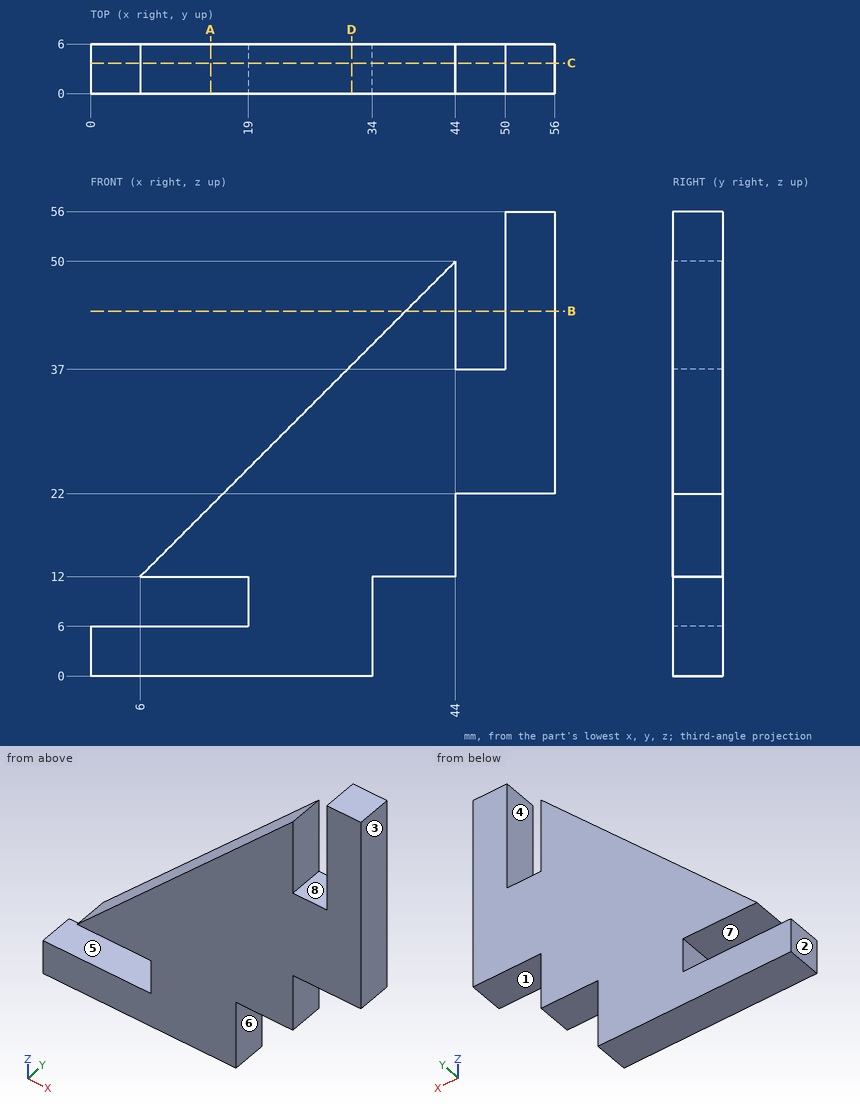
Print and shaded views of the part. All mm, measured from the part's lowest x, y and z. A direction names the side the tool comes from. Coordinates: 2 decimals unless noted, no trailing zeros. Loops run counter-clockwise (first coordinate to the right, second up) from the corner with the lowest first, then second, coordinate; pieces in that order, holes last. Notation, with made-up numbers: (87, 66) - (137, 66) arc R17 ccw to (137, 97) - close; hole circle Ø9 at (72, 30.5). An arc over 180 degrees is marked (long way). Write item = value, one per line. Start each with the question number.
Item 1: Flat gauge pins, fed straight in: pin 1 Ø1.8 at (y, z) = (1.5, 10.5) entering from -X; pin 2 Ø1.8 at (x, y) = (50.5, 4) entering from -Z; pin 3 Ø1.8 at (y, z) = (1.5, 6.5) entering from +X. Where does each tip first touch, or does it go through?
Item 2: Mould opens along X. For the marked faces 6, 7 and 8 say: released by +X, released by -X, zero draft, split by the parting line, or undercut.
Item 3: Cut at B-B, the plane z = 44. Give the cut face in (x, y), and give its area (3 significant figures).
Item 4: Cut at D-D, the plane x = 31.5. Give the cut face in (y, z).
Item 5: Wall check: L1, parallel to Z at x = 46, y = 4.85; L2, parallel to X at y = 3.95, z = 52.5; L3, parallel to X at y = 0.5, z = 6.5. Give the ranges that are in metal, low to high. Write a range as from..to.
Item 6: Cut at A-A, the plane x = 14.5. Give the cut face in (y, z).
Item 7: Cut at C-C, the plane y = 3.7. Give the cut face in (x, z).
Item 8: 3-axis set-ups, long thin cutter, end or side, ignore diameter. For the marked faces 1, 2, 3, 4 and 5: which of +Z, -Z, +X, -X, +Y, -Y reach the whole face in a straight line?
The answers:
q1.pin_1 = 19
q1.pin_2 = 22
q1.pin_3 = 34
q2.face_6 = released by +X
q2.face_7 = zero draft
q2.face_8 = undercut
q3.outline = (38, 0) - (44, 0) - (44, 6) - (38, 6) - close; (50, 0) - (56, 0) - (56, 6) - (50, 6) - close
q3.area = 72.0 mm2
q4.outline = (0, 0) - (6, 0) - (6, 37.5) - (0, 37.5) - close
q5.L1 = 22..37
q5.L2 = 50..56
q5.L3 = 19..34
q6.outline = (0, 0) - (6, 0) - (6, 6) - (0, 6) - close; (0, 12) - (6, 12) - (6, 20.5) - (0, 20.5) - close
q7.outline = (0, 0) - (34, 0) - (34, 12) - (44, 12) - (44, 22) - (56, 22) - (56, 56) - (50, 56) - (50, 37) - (44, 37) - (44, 50) - (6, 12) - (19, 12) - (19, 6) - (0, 6) - close
q8.face_1 = -Z, +X, +Y, -Y
q8.face_2 = +Z, -Z, -X, +Y, -Y
q8.face_3 = +Z, -Z, +X, +Y, -Y
q8.face_4 = +Z, +Y, -Y
q8.face_5 = -X, +Y, -Y
